from build123d import *

# Parameters (mm, degrees)
F0_W     = 7.26223737
F0_H     = 14.0403658152
F0_H_2   = 16.6169349104
F0_W_2   = 21.9669826329
F0_W_3   = 15.7987792045
F0_W_4   = 12.2116522557
F0_H_3   = 15.2750127017
F1_DEPTH = 2.54
F2_T     = -0.508


with BuildPart() as f1:
    # F0 (on Top) → F1 (new body)
    with BuildSketch(Plane.XY):
        Polygon((-48.5124173612, 7.03542912), (-20.8847596319, 7.03542912), (22.3510192425, 35.0815849379), (-20.8847596319, 63.1277407557), (-48.5124173612, 63.1277407557), (-48.5124173612, 57.2236290348), (-60.9962199777, 57.2236290348), (-60.9962199777, 63.1277407557), (-91.6035394222, 63.1277407557), (-91.6035394222, 7.03542912), (-60.9962199777, 7.03542912), (-60.9962199777, 13.134556353), (-48.5124173612, 13.134556353), align=None)
        with Locations((-85.432421416, 16.5956113487)):
            Rectangle(F0_W, F0_H, mode=Mode.SUBTRACT)
        Polygon((-57.2943203151, 15.6745556742), (-63.5362192988, 15.6745556742), (-63.5362192988, 9.5754284412), (-79.261302948, 9.5754284412), (-79.261302948, 23.6157942563), (-57.2943203151, 23.6157942563), align=None, mode=Mode.SUBTRACT)
        Polygon((-38.955539465, 9.5754284412), (-45.97241804, 9.5754284412), (-45.97241804, 15.6745556742), (-54.7543186694, 15.6745556742), (-54.7543186694, 23.6157942563), (-38.955539465, 23.6157942563), align=None, mode=Mode.SUBTRACT)
        with Locations((-85.432421416, 34.4642614946)):
            Rectangle(F0_W, F0_H_2, mode=Mode.SUBTRACT)
        with Locations((-68.2778116316, 34.4642614946)):
            Rectangle(F0_W_2, F0_H_2, mode=Mode.SUBTRACT)
        with Locations((-46.8549290672, 34.4642614946)):
            Rectangle(F0_W_3, F0_H_2, mode=Mode.SUBTRACT)
        with Locations((-30.3097135541, 16.5956113487)):
            Rectangle(F0_W_4, F0_H, mode=Mode.SUBTRACT)
        with Locations((-30.3097135541, 34.4642614946)):
            Rectangle(F0_W_4, F0_H_2, mode=Mode.SUBTRACT)
        Polygon((-7.5185770554, 18.7333902767), (-21.6364338994, 9.5754284412), (-21.6638874263, 9.5754284412), (-21.6638874263, 23.6157942563), (-21.6638874263, 26.1557940394), (-21.6638874263, 42.7727289498), (-21.6638874263, 45.3127287328), (-21.6638874263, 60.5877414346), (-21.6364338994, 60.5877414346), (-7.5185770554, 51.429779599), align=None, mode=Mode.SUBTRACT)
        with Locations((-85.432421416, 52.9502350837)):
            Rectangle(F0_W, F0_H_3, mode=Mode.SUBTRACT)
        Polygon((-79.261302948, 60.5877414346), (-63.5362192988, 60.5877414346), (-63.5362192988, 54.6836297136), (-57.2943203151, 54.6836297136), (-57.2943203151, 45.3127287328), (-79.261302948, 45.3127287328), align=None, mode=Mode.SUBTRACT)
        Polygon((-54.7543186694, 54.6836297136), (-45.97241804, 54.6836297136), (-45.97241804, 60.5877414346), (-38.955539465, 60.5877414346), (-38.955539465, 45.3127287328), (-54.7543186694, 45.3127287328), align=None, mode=Mode.SUBTRACT)
        Polygon((-4.9785770554, 49.7821341158), (17.6836978644, 35.0815849379), (-4.9785770554, 20.38103576), align=None, mode=Mode.SUBTRACT)
        with Locations((-30.3097135541, 52.9502350837)):
            Rectangle(F0_W_4, F0_H_3, mode=Mode.SUBTRACT)
    extrude(amount=F1_DEPTH)

    # F2
    f2_openings = [f1.faces().sort_by_distance(p)[0] for p in [
        (-90.333422, 35.081585, 2.54),
    ]]
    offset(amount=F2_T, openings=f2_openings, kind=Kind.INTERSECTION)


solid = f1.part
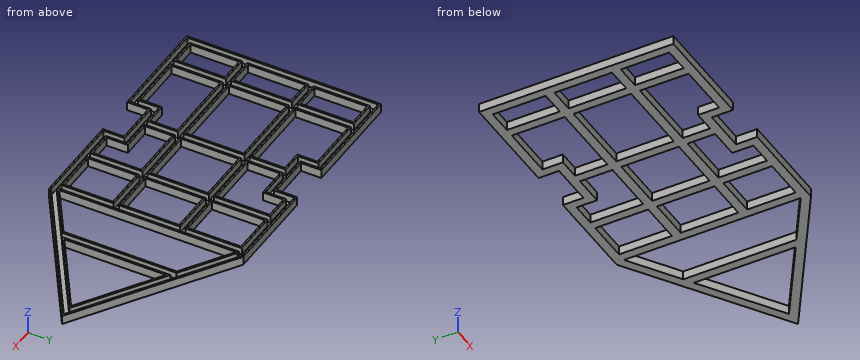
Could you check a few things on this model? Use its own coordinates, in mm. Give positions to 0.01 mm unless a question says otherwise; leave off trailing zeros. Order: outer loops, then holes, each group sorted by start corner. A loop starts at its lowest first (then second) coordinate and runs counter-clockwise, first axis right, second up.
1. Suppose I cut it at C-C (x = -15). Write out the boundary of the cut face in (y, z).
Answers below:
outline: (10.85, 0) - (13.88, 0) - (13.88, 2.54) - (13.27, 2.54) - (13.27, 0.51) - (11.46, 0.51) - (11.46, 2.54) - (10.85, 2.54) - close; (56.28, 0) - (59.31, 0) - (59.31, 2.54) - (58.7, 2.54) - (58.7, 0.51) - (56.89, 0.51) - (56.89, 2.54) - (56.28, 2.54) - close
2. I need wall thicknesses on L1, parallel to Y at x = -65, z = 0.25; L2, parallel to Y at x = 10, z = 0.7; L3, parallel to X at y = 56.5, z = 0.45. Which ranges of each line are inside material? Lowest first, please.
Answers below:
L1: y = 7.04 to 9.58, 23.62 to 26.16, 42.77 to 45.31, 60.59 to 63.13
L2: y = 27.07 to 27.68, 29.49 to 30.1, 40.07 to 40.67, 42.49 to 43.09
L3: x = -91.6 to -89.06, -81.8 to -79.26, -63.54 to -45.97, -38.96 to -36.42, -24.2 to -21.66, -15.33 to -10.67
3. For pin 1 (10 mm diameter, centred on x = -40, y = 25.5, fed in from -Z); pin 2 (1 mm diameter, centred on x = -11, z = 2, fed in from -Y); pin 3 (1.3 mm diameter, centred on y = 18, z = 2, fed in from +X), each with a flat end and sliding along its axis, tell me the tip position at first contact or that it passes through.
Answers below:
pin 1: stops at z = 0
pin 2: stops at y = 13.12
pin 3: stops at x = -2.98
4. Suppose I cut it at A-A (x = -34.5). State how many separate pieces and enclosed holes the cut face has, plus the area to 3 significant figures.
Answers below:
separate pieces: 4
enclosed holes: 0
area: 13.4 mm2
